Geometry check sheet. Reference: the model listing, model coordinates, mm. Face numbers are marked on the shaded views. A direction names the side the tool comes from. Give positions to 0.01 mm unless a question says otherwise; leave off trailing zeros. Loops run counter-clockwise (first coordinate to the right, second up) from the corner with the lowest first, then second, coordinate; pieces in that order, holes last. Notation, with made-up numbers: (86, -5) -> (128, -5) arc R17 ccw to (128, 8) -> close; hole circle Ø11 at (38, 29.25). An arc over 180 degrees is marked (long way). Write each question's results on one line, items separated by ' | '. Start each with the question number.
1) Set-up check for the marked faces 1, 2 and 3: record each of +Z, -Z, +X, -X, +Y, -Y from which the full face is reachable in a straight line by a thin tool's end or side.
2) Draft check along Z on the marked faces 4, 5, 6 and 7. Enter one of: pulls with the +Z half, pulls with the -Z half, needs draft (parallel to the pull), parting line crosses it, or undercut.
3) Sectioned sample at D-D on z = 20. Record the cut outline in (x, y).
4) Sectioned sample at C-C on z = -1. Record the cut outline in (x, y), then the cut area to 3 significant figures.
5) Sectioned sample at A-A on y = -6.5. Record the cut outline in (x, z), then the cut area to 4 significant figures.
6) Scan lines: line 1 (X direction, y = 3.5, z = -0.5); line 2 (Z direction, x = -9.5, y = 2.75); line 3 (Y direction, x = -11.5, z = 1). Record each from-to range of solid material in increasing order. Write a range as from..to.
7) Depth check by flat-ended pin: pin 1 (1 mm diameter, centred on y = 3, z = 0, fed in from -X); pin 2 (3 mm diameter, centred on x = 6, z = 6, fed in from +Y); pin 3 (3 mm diameter, centred on x = 16, y = -6, fed in from -Z). Enter the tip coordinate at first touch or a pass-through.
8) Sectioned sample at B-B on x = -1.5. Record the cut outline in (y, z).
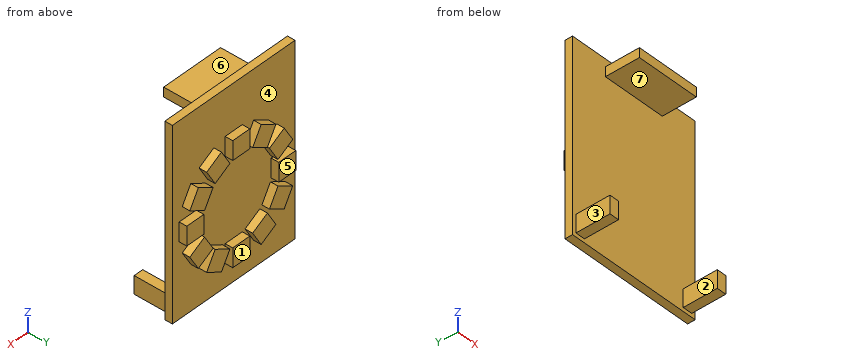
```python
from build123d import *

# Parameters (mm, degrees)
SKETCH1_W           = 36
SKETCH1_H           = 50
BOSS_EXTRUDE1_DEPTH = 2
SKETCH2_W           = 5
SKETCH2_H           = 5
BOSS_EXTRUDE2_DEPTH = 2
CIRPATTERN1_COUNT   = 12
SKETCH3_W           = 16.7
SKETCH3_H           = 2.5
SKETCH3_W_2         = 2.5
SKETCH3_H_2         = 4.7
BOSS_EXTRUDE3_DEPTH = 9


with BuildPart() as part:
    # Sketch1 → Boss-Extrude1 (new body)
    with BuildSketch(Plane(origin=(0, 0, 0), x_dir=(1, 0, 0), z_dir=(0, 1, 0))):
        with Locations((0, -3)):
            Rectangle(SKETCH1_W, SKETCH1_H)
    extrude(amount=BOSS_EXTRUDE1_DEPTH)

    # Sketch2 → Boss-Extrude2 (add)
    with BuildSketch(Plane(origin=(0, 2, 0), x_dir=(1, 0, 0), z_dir=(0, 1, 0))):
        with Locations((0, 13.5)):
            Rectangle(SKETCH2_W, SKETCH2_H)
    boss_extrude2 = extrude(amount=BOSS_EXTRUDE2_DEPTH)

    # CirPattern1: Boss-Extrude2 ×12 about axis
    cirpattern1_axis = Axis((0, 0, 0), (0, 1, 0))
    for i in range(1, CIRPATTERN1_COUNT):
        add(boss_extrude2.rotate(cirpattern1_axis, i * 360 / CIRPATTERN1_COUNT))

    # Sketch3 → Boss-Extrude3 (add)
    with BuildSketch(Plane.XZ):
        with Locations((0, 24.75)):
            Rectangle(SKETCH3_W, SKETCH3_H)
        with Locations((-15.75, -18.65)):
            Rectangle(SKETCH3_W_2, SKETCH3_H_2)
        with Locations((15.75, -18.65)):
            Rectangle(SKETCH3_W_2, SKETCH3_H_2)
    extrude(amount=BOSS_EXTRUDE3_DEPTH)


solid = part.part
```
Result:
1) face 1: +Z, -Z, +X, -X, +Y | face 2: +Z, -Z, -Y | face 3: +Z, -Z, -X, -Y
2) face 4: undercut | face 5: needs draft | face 6: pulls with the +Z half | face 7: pulls with the -Z half
3) outline: (-18, 0) -> (18, 0) -> (18, 2) -> (-18, 2) -> close
4) outline: (-18, 0) -> (18, 0) -> (18, 2) -> (16, 2) -> (16, 4) -> (11, 4) -> (11, 2) -> (-11, 2) -> (-11, 4) -> (-16, 4) -> (-16, 2) -> (-18, 2) -> close | area: 92.0 mm^2
5) outline: (-17, -21) -> (-14.5, -21) -> (-14.5, -16.3) -> (-17, -16.3) -> close; (-8.35, 23.5) -> (8.35, 23.5) -> (8.35, 26) -> (-8.35, 26) -> close; (14.5, -21) -> (17, -21) -> (17, -16.3) -> (14.5, -16.3) -> close | area: 65.25 mm^2
6) line 1: -16..-11, 11..16 | line 2: -12.99..-11.45, -8.37..-5.55, 5.55..8.37, 11.45..12.99 | line 3: 0..4
7) pin 1: x = -16 | pin 2: y = 2 | pin 3: z = -21
8) outline: (-9, 23.5) -> (0, 23.5) -> (0, -22) -> (2, -22) -> (2, -16) -> (4, -16) -> (4, -11) -> (2, -11) -> (2, 11) -> (4, 11) -> (4, 16) -> (2, 16) -> (2, 28) -> (0, 28) -> (0, 26) -> (-9, 26) -> close
